Can you work these out from the drawing? Everything is in mm from the part's minimum corner. Coordinates: 2 decimals unless noted, no trailing zeros. Order: outer loops, then holes, each group sorted by start corner. A loop starts at its lowest first (then second) coordinate and runs counter-clockwise, first axis right, second up. Notation, with made-up numbers: (84.5, -23) - (89.5, -23) arc R24 cw to (89.5, -1) - close; hole circle Ø10 at (23, -31). An arc over 180 degrees is marked (long way). Use a Markdown table: item, result. Add a question column.
(1) I want a section at A-A (y = 2.15). List the corners of the cut face in (x, z) for me.
(2) I want a section at C-C (x = 74.5). List the corners of the cut face in (y, z) for me.
(3) If I drill on L1, parallel to Z at x = 150, y = 1.45; L2, parallel to Z at x = 25, y = 3.9; L3, parallel to Z at x = 14.5, y = 3.7, over which ranges is the centre line in solid material (lowest first)? Write a range as [from, to].
(4) I want a section at B-B (z = 68.5). List the corners of the cut face in (x, y) for me, and give its area (3 significant figures).
(5) For pin 1 Ø1.5 at (x, y) = (239, 3.5) entering from -Z; pin 2 Ø2.5 at (y, z) = (2.5, 13) entering from -X; pin 3 Ø2.5 at (x, y) = (259.5, 3.5) entering from +Z, each with a flat end and sliding along its axis, tell me the tip position at first contact or that it passes through.
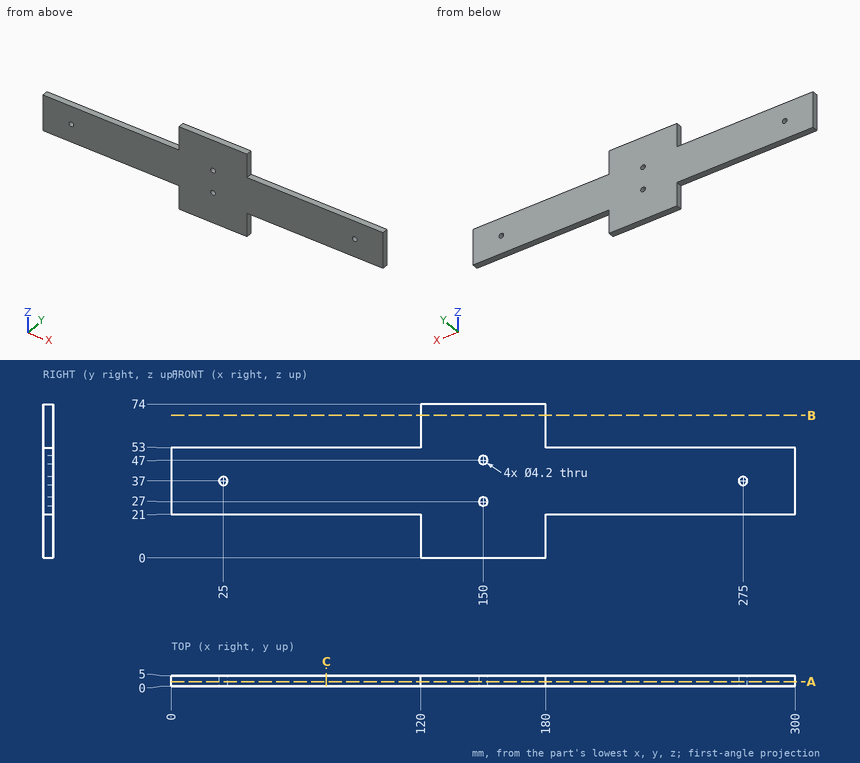
Answers follow:
| question | item | result |
|---|---|---|
| 1 | outline | (0, 21) - (120, 21) - (120, 0) - (180, 0) - (180, 21) - (300, 21) - (300, 53) - (180, 53) - (180, 74) - (120, 74) - (120, 53) - (0, 53) - close; hole circle Ø4.2 at (25, 37); hole circle Ø4.2 at (150, 27); hole circle Ø4.2 at (150, 47); hole circle Ø4.2 at (275, 37) |
| 2 | outline | (0, 21) - (5, 21) - (5, 53) - (0, 53) - close |
| 3 | L1 | z = [0, 24.9], [29.1, 44.9], [49.1, 74] |
| 3 | L2 | z = [21, 34.9], [39.1, 53] |
| 3 | L3 | z = [21, 53] |
| 4 | outline | (120, 0) - (180, 0) - (180, 5) - (120, 5) - close |
| 4 | area | 300 mm² |
| 5 | pin 1 | stops at z = 21 |
| 5 | pin 2 | stops at x = 120 |
| 5 | pin 3 | stops at z = 53 |
